For this review, use the dimensioned drawing (mm, ordinates from the lowest corner) and the shaded views. Coordinates: 2 decimals unless noted, no trailing zeros. Loops run counter-clockwise (first coordinate to the right, second up) from the corner with the lowest first, then second, coordinate; pieces in that order, holes last.
1. Take a section at B-B, the plane y = 2.5. State the section outline as (x, z) points.
2. Take a section at C-C, the plane z = 1.8. State the section outline as (x, y) points, then the cut area to 3 significant figures.
3. Mouldability with a two-part tool opening along Y and no side actions: class the marked faces 1, 2 and 3 as pulls with the +Y half, pulls with the -Y half, needs draft (parallel to the pull), parting line crosses it, or undercut.
4. Clearance check with a flat-ended pin moving along its axis: P1, Ø2, axis at x = 6.5, y = 2.5, coming from the -Z side. State where the tip first meets the part, or that it passes through.
5. Take a section at A-A, the plane x = 6.5. State the section outline as (y, z) points, then the cut area to 4 significant figures.
6. To check wall thickness, follow probe 1 along Y at (x, z) = (23.5, 2.3); probe 2 along X at (y, z) = (3.25, 0.3); probe 3 along X at (y, z) = (2.05, 0.25). State the ranges of each line that lie inside material, in increasing order.
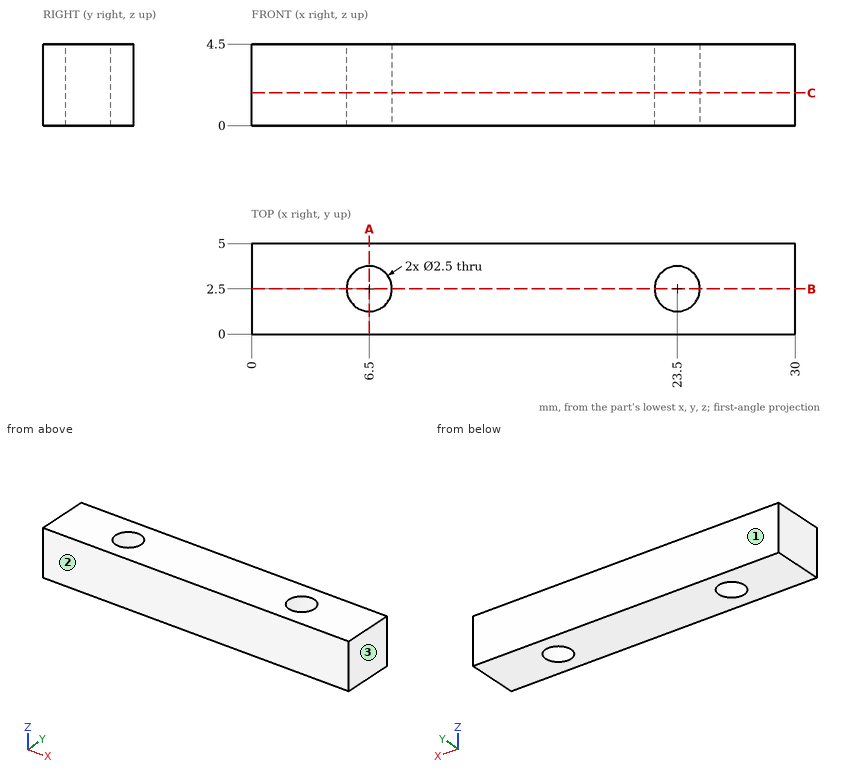
Results list:
1. outline: (0, 0) - (5.25, 0) - (5.25, 4.5) - (0, 4.5) - close; (7.75, 0) - (22.25, 0) - (22.25, 4.5) - (7.75, 4.5) - close; (24.75, 0) - (30, 0) - (30, 4.5) - (24.75, 4.5) - close
2. outline: (0, 0) - (30, 0) - (30, 5) - (0, 5) - close; hole circle Ø2.5 at (6.5, 2.5); hole circle Ø2.5 at (23.5, 2.5)
2. area: 140 mm2
3. face 1: pulls with the +Y half
3. face 2: pulls with the -Y half
3. face 3: needs draft
4. P1: passes through
5. outline: (0, 0) - (1.25, 0) - (1.25, 4.5) - (0, 4.5) - close; (3.75, 0) - (5, 0) - (5, 4.5) - (3.75, 4.5) - close
5. area: 11.25 mm2
6. probe 1: y = 0 to 1.25, 3.75 to 5
6. probe 2: x = 0 to 5.5, 7.5 to 22.5, 24.5 to 30
6. probe 3: x = 0 to 5.33, 7.67 to 22.33, 24.67 to 30
